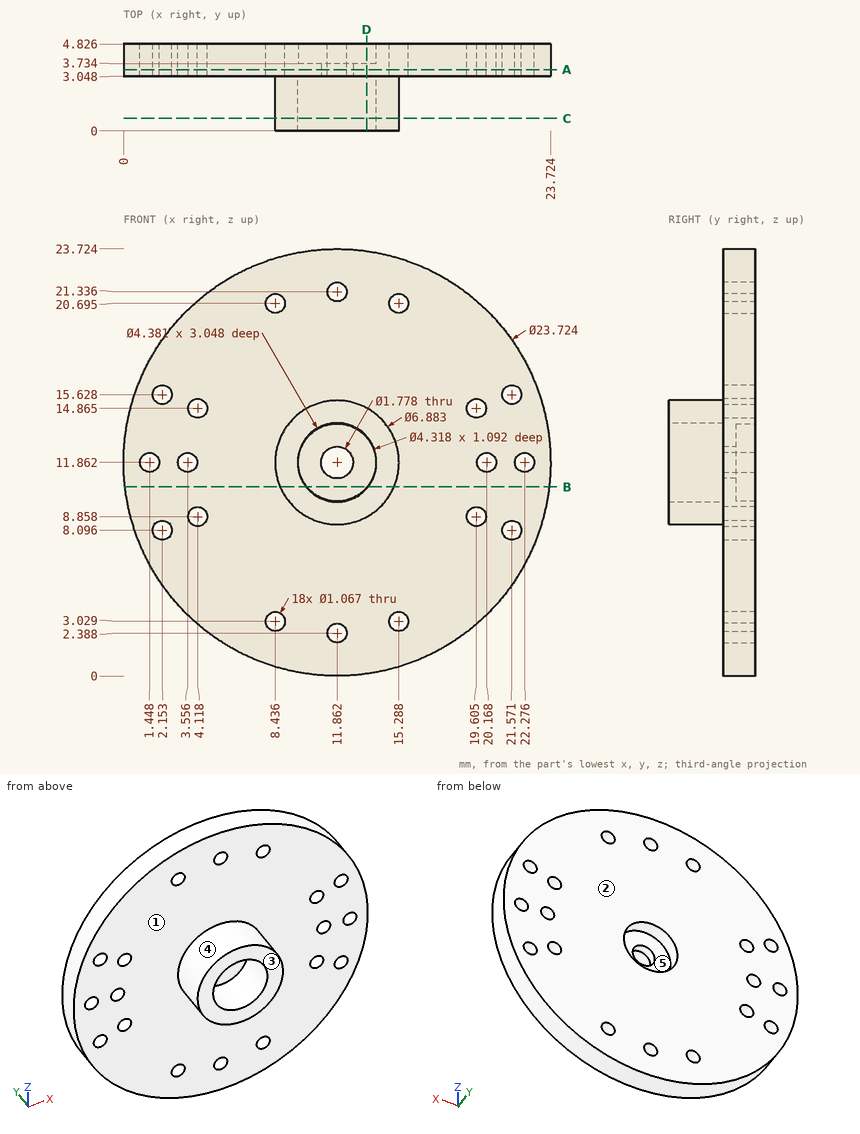
Print and shaded views of the part. All mm, measured from the part's lowest x, y and z. A direction names the side the tool comes from. Coordinates: 2 decimals unless noted, no trailing zeros. Order: outer loops, then holes, each group sorted by start corner. A loop starts at its lowest first (then second) coordinate and runs counter-clockwise, first axis right, second up. Notation, with made-up numbers: (87, 7.5) - (118, 7.5) arc R25 cw to (118, 35.5) - close; hole circle Ø11 at (-1, 83.25). An arc over 180 degrees is marked (long way). Return JSON: item names as keys, results as strings. Group by question number.
Item 1: Cut at A-A (y = 3.4). State how many separate pieces and enclosed holes the cut face has.
Item 2: Which spindle directions (+Z, -Z, +X, -X, +Y, -Y) get a long thin tool onto all of the face, cutting with end or side? Do the marked faces 1 and 2. Say none if no direction does.
Item 3: Cut at C-C (y = 0.7). List the corners of the cut face in (x, z).
Item 4: Cut at B-B (z = 10.5). List the corners of the cut face in (x, y) (1 decimal).
Item 5: Pull direction X, two halves, no side cores. Call the marked faces 3, 4 and 5: pulls with the +X half, pulls with the -X half, needs draft (parallel to the pull), parting line crosses it, or undercut.
Item 6: Pin check, flat tips, straight feed: pin 1 (2.5 mm diameter, centred on x = 11.86, z = 11.86, fed in from +Y); pin 2 (2 mm diameter, centred on y = 4, z = 14, fed in from +X); pin 3 (3 mm diameter, centred on x = 12.5, z = 4, fed in from -Y). Stop position of each tip, or through.
Item 7: Cut at D-D (x = 13.5). List the corners of the cut face in (y, z) (1 decimal).
Item 8: Drill centre lines: probe 1 along X at (y, z) = (3.9, 15.5) (1 decimal); probe 2 along Y at (x, z) = (7.25, 2.75) (1 decimal); probe 3 along Y at (x, z) = (13.75, 11.5). Where is each one in solid material? Low to high. Write a range as from..to.
Check values:
{
 "1": {"separate pieces": "1", "enclosed holes": "19"},
 "2": {"face 1": "-Y", "face 2": "+Z, -Z, +X, -X, +Y"},
 "3": {"outline": "circle Ø6.88 at (11.86, 11.86); hole circle Ø4.38 at (11.86, 11.86)"},
 "4": {"outline": "(0.1, 3) - (8.7, 3) - (8.7, 0) - (10.1, 0) - (10.1, 3) - (13.6, 3) - (13.6, 0) - (15, 0) - (15, 3) - (23.6, 3) - (23.6, 4.8) - (13.5, 4.8) - (13.5, 3.7) - (10.2, 3.7) - (10.2, 4.8) - (0.1, 4.8) - close"},
 "5": {"face 3": "needs draft", "face 4": "parting line crosses it", "face 5": "undercut"},
 "6": {"pin 1": "stops at y = 3.73", "pin 2": "stops at x = 23.67", "pin 3": "stops at y = 3.05"},
 "7": {"outline": "(0, 8.8) - (3, 8.8) - (3, 0.1) - (4.8, 0.1) - (4.8, 10.5) - (3.7, 10.5) - (3.7, 13.3) - (4.8, 13.3) - (4.8, 23.6) - (3, 23.6) - (3, 14.9) - (0, 14.9) - (0, 13.3) - (3, 13.3) - (3, 10.4) - (0, 10.4) - close"},
 "8": {"probe 1": "x = 0.6..1.6, 2.7..21.1, 22.1..23.2", "probe 2": "y = 3..4.8", "probe 3": "y = 3.05..3.73"}
}
